The figure shows three views and two pictorial views of one solid part (mm, origin at its lowest corner). Answer the questions. Coordinates: 2 decimals unless noted, no trailing zeros. Loops run counter-clockwise (first coordinate to the right, second up) from the corner with the lowest first, then second, coordinate; pieces in that order, holes last. Notation, with made-up numbers: (18, -16) - (53, -16) arc R32 cw to (53, 11) - close; hole circle Ø7 at (-10.5, 86). An arc over 180 degrees is marked (long way). Return JSON: item names as keys, results as strings. Group by question number.
1. The mould has two halves that part along Y. Classify the marked faces 1, 2 and 3: pulls with the +Y half, pulls with the -Y half, needs draft (parallel to the pull), parting line crosses it, or undercut.
2. Find the intervals of material crossed by line 1 along Y through (x, z) = (30.5, 0.7); line 2 along X through (y, z) = (21.5, 0.45); line 3 along Z through (x, y) = (8, 27) (1 decimal), in increasing order.
3. Section A-A (x = 20.5) is taken. Write down the section's boundary in (y, z) (1 decimal).
4. Section B-B (z = 1.15) is taken. Write down the section's boundary in (x, y).
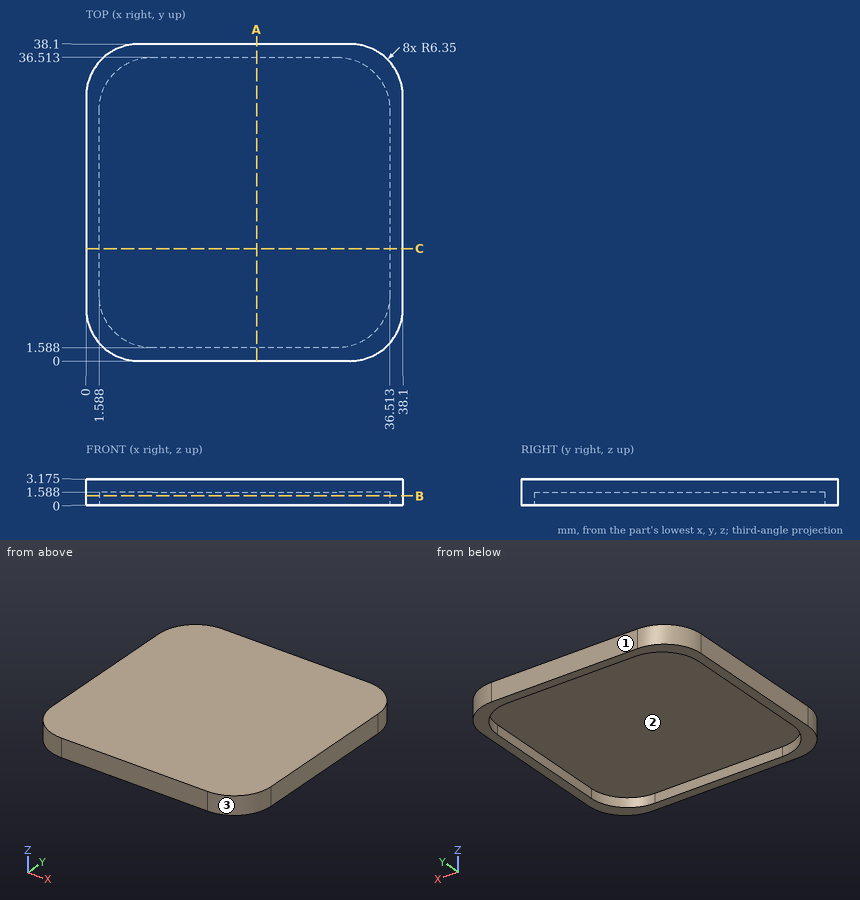
The answers:
{
 "1": {"face 1": "pulls with the +Y half", "face 2": "undercut", "face 3": "pulls with the -Y half"},
 "2": {"line 1": "y = 0 to 1.6, 36.5 to 38.1", "line 2": "x = 0 to 1.59, 36.51 to 38.1", "line 3": "z = 1.6 to 3.2"},
 "3": {"outline": "(0, 0) - (1.6, 0) - (1.6, 1.6) - (36.5, 1.6) - (36.5, 0) - (38.1, 0) - (38.1, 3.2) - (0, 3.2) - close"},
 "4": {"outline": "(0, 6.35) arc R6.35 ccw to (6.35, 0) - (31.75, 0) arc R6.35 ccw to (38.1, 6.35) - (38.1, 31.75) arc R6.35 ccw to (31.75, 38.1) - (6.35, 38.1) arc R6.35 ccw to (0, 31.75) - close; hole (1.59, 7.94) arc R6.35 ccw to (7.94, 1.59) - (30.16, 1.59) arc R6.35 ccw to (36.51, 7.94) - (36.51, 30.16) arc R6.35 ccw to (30.16, 36.51) - (7.94, 36.51) arc R6.35 ccw to (1.59, 30.16) - close"}
}
